from build123d import *

# Parameters (mm, degrees)
CUT_EXTRUDE2_REACH = 103.6
SKETCH3_R          = 3.175
FILLET1_R          = 3.175
FILLET2_R          = 1.5875


with BuildPart() as part:
    # Sketch1 → Revolve1 (revolve)
    with BuildSketch(Plane.XY):
        Polygon((-12.7, 9.525), (-30.109602918, 39.679316793), (-30.109602918, 50.8), (-30.109602918, 69.85), (-11.059602918, 69.85), (-11.059602918, 50.8), (71.490397082, 50.8), (0, 9.525), align=None)
    revolve(axis=Axis((0, 0, 0), (1, 0, 0)))

    # Sketch3 → Cut-Extrude2 (cut, up to next)
    with BuildSketch(Plane.ZY.offset(30.109602918), mode=Mode.PRIVATE) as cut_extrude2_sk1:
        with Locations((0, 59.9186)):
            Circle(SKETCH3_R)
    cut_extrude2_tool1 = extrude(cut_extrude2_sk1.sketch, amount=-CUT_EXTRUDE2_REACH, mode=Mode.PRIVATE) & part.part
    add(cut_extrude2_tool1.solids().sort_by_distance((-30.109603, 59.9186, 0))[0], mode=Mode.SUBTRACT)
    # Sketch3 → Cut-Extrude2 (cut, up to next)
    with BuildSketch(Plane.ZY.offset(30.109602918), mode=Mode.PRIVATE) as cut_extrude2_sk2:
        with Locations((42.368848379, 42.368848379)):
            Circle(SKETCH3_R)
    cut_extrude2_tool2 = extrude(cut_extrude2_sk2.sketch, amount=-CUT_EXTRUDE2_REACH, mode=Mode.PRIVATE) & part.part
    add(cut_extrude2_tool2.solids().sort_by_distance((-30.109603, 42.368848, 42.368848))[0], mode=Mode.SUBTRACT)
    # Sketch3 → Cut-Extrude2 (cut, up to next)
    with BuildSketch(Plane.ZY.offset(30.109602918), mode=Mode.PRIVATE) as cut_extrude2_sk3:
        with Locations((59.9186, 0)):
            Circle(SKETCH3_R)
    cut_extrude2_tool3 = extrude(cut_extrude2_sk3.sketch, amount=-CUT_EXTRUDE2_REACH, mode=Mode.PRIVATE) & part.part
    add(cut_extrude2_tool3.solids().sort_by_distance((-30.109603, 0, 59.9186))[0], mode=Mode.SUBTRACT)
    # Sketch3 → Cut-Extrude2 (cut, up to next)
    with BuildSketch(Plane.ZY.offset(30.109602918), mode=Mode.PRIVATE) as cut_extrude2_sk4:
        with Locations((42.368848379, -42.368848379)):
            Circle(SKETCH3_R)
    cut_extrude2_tool4 = extrude(cut_extrude2_sk4.sketch, amount=-CUT_EXTRUDE2_REACH, mode=Mode.PRIVATE) & part.part
    add(cut_extrude2_tool4.solids().sort_by_distance((-30.109603, -42.368848, 42.368848))[0], mode=Mode.SUBTRACT)
    # Sketch3 → Cut-Extrude2 (cut, up to next)
    with BuildSketch(Plane.ZY.offset(30.109602918), mode=Mode.PRIVATE) as cut_extrude2_sk5:
        with Locations((0, -59.9186)):
            Circle(SKETCH3_R)
    cut_extrude2_tool5 = extrude(cut_extrude2_sk5.sketch, amount=-CUT_EXTRUDE2_REACH, mode=Mode.PRIVATE) & part.part
    add(cut_extrude2_tool5.solids().sort_by_distance((-30.109603, -59.9186, 0))[0], mode=Mode.SUBTRACT)
    # Sketch3 → Cut-Extrude2 (cut, up to next)
    with BuildSketch(Plane.ZY.offset(30.109602918), mode=Mode.PRIVATE) as cut_extrude2_sk6:
        with Locations((-42.368848379, -42.368848379)):
            Circle(SKETCH3_R)
    cut_extrude2_tool6 = extrude(cut_extrude2_sk6.sketch, amount=-CUT_EXTRUDE2_REACH, mode=Mode.PRIVATE) & part.part
    add(cut_extrude2_tool6.solids().sort_by_distance((-30.109603, -42.368848, -42.368848))[0], mode=Mode.SUBTRACT)
    # Sketch3 → Cut-Extrude2 (cut, up to next)
    with BuildSketch(Plane.ZY.offset(30.109602918), mode=Mode.PRIVATE) as cut_extrude2_sk7:
        with Locations((-59.9186, 0)):
            Circle(SKETCH3_R)
    cut_extrude2_tool7 = extrude(cut_extrude2_sk7.sketch, amount=-CUT_EXTRUDE2_REACH, mode=Mode.PRIVATE) & part.part
    add(cut_extrude2_tool7.solids().sort_by_distance((-30.109603, 0, -59.9186))[0], mode=Mode.SUBTRACT)
    # Sketch3 → Cut-Extrude2 (cut, up to next)
    with BuildSketch(Plane.ZY.offset(30.109602918), mode=Mode.PRIVATE) as cut_extrude2_sk8:
        with Locations((-42.368848379, 42.368848379)):
            Circle(SKETCH3_R)
    cut_extrude2_tool8 = extrude(cut_extrude2_sk8.sketch, amount=-CUT_EXTRUDE2_REACH, mode=Mode.PRIVATE) & part.part
    add(cut_extrude2_tool8.solids().sort_by_distance((-30.109603, 42.368848, -42.368848))[0], mode=Mode.SUBTRACT)

    # Fillet1
    fillet1_edges = [part.edges().sort_by_distance(p)[0] for p in [
        (0, -9.525, 0),
        (-12.7, -9.525, 0),
    ]]
    fillet(fillet1_edges, radius=FILLET1_R)

    # Fillet2
    fillet2_edges = [part.edges().sort_by_distance(p)[0] for p in [
        (-11.059602918, -50.8, 0),
    ]]
    fillet(fillet2_edges, radius=FILLET2_R)


solid = part.part
The model under review builds one solid part; all positions refer to its coordinate system, in mm. A direction names the side the tool comes from. Coordinates: 2 decimals unless noted, no trailing zeros. Write each loop counter-clockwise with the first axis right and the second up, starting at its lowest first coordinate (ties: lowest second). Pieces come first, ordered by that corner, then holes. Notation, with made-up numbers: (-15, 18.5) - (-5, 18.5) arc R34 cw to (-5, 57.5) - close; hole circle Ø7 at (28, 87). An arc over 180 degrees is marked (long way). Answer as a JSON object with one key per item and string values. Group by question number.
1. Machinability: for faces 5 (the face through (-20.718, 45.046, 44.076)), 6 (the face through (-11.06, 15, -51)), which of the approach directions +Z, -Z, +X, -X, +Y, -Y give a long, thin tool a straight path to every point of the face, cutting with its end or side? Answer none if there is none.
2. Add section A-A (y = 0). Give the number of separate pieces and of enclosed holes in the cut face, plus the area to 3 significant figures.
3. Add section C-C (x = 14.5). Give the boundary of the cut face in (y, z).
4. Mouldability with a two-part tool opening along Z and no side actions: class faces 1 (the face through (-20.718, -63.018, -0.688)), 2 (the face through (-30.11, 30, -30)), 3 (the face through (-20.451, -55.431, -42.503)), 4 (the face through (-20.72, -44.3, -44.89)) as pulls with the +Z half, pulls with the -Z half, needs draft (parallel to the pull), parting line crosses it, or undercut.
5. Clearance check with flat-ended pins moving along their axes: pin 1 Ø10 at (x, y) = (23, -51.5) entering from +Z; pin 2 Ø10 at (y, z) = (-42.37, -42.37) entering from +X; pin 3 Ø5 at (y, z) = (-42.37, 42.37) entering from +X; pin 4 Ø1 at (x, y) = (-5.5, 2.5) entering from +Z. State where each tip first meets the part, or that it passes through.
6. To check wall thickness, follow probe 1 along Z at (x, y) = (-4, 0) (3 decimals); probe 2 along X at (y, z) = (48, 34); probe 3 along Z at (x, y) = (48, 1.5). State the ranges of each line that lie inside material, in increasing order.
Findings:
{
 "1": {"face 5": "+X, -X", "face 6": "+X"},
 "2": {"separate pieces": "4", "enclosed holes": "0", "area": "5,400 mm²"},
 "3": {"outline": "circle Ø101.6 at (0, 0); hole circle Ø35.79 at (0, 0)"},
 "4": {"face 1": "undercut", "face 2": "needs draft", "face 3": "parting line crosses it", "face 4": "undercut"},
 "5": {"pin 1": "z = 20.45", "pin 2": "x = -11.06", "pin 3": "through", "pin 4": "z = 50.76"},
 "6": {"probe 1": "-50.8 to -9.525, 9.525 to 50.8", "probe 2": "-30.11 to -11.06", "probe 3": "-50.78 to -37.21, 37.21 to 50.78"}
}
